Design review of the part built by this model. Coordinates are the model's own, in mm. A direction names the side the tool comes from. Round coordinates to 2 decimals unless told otherwise and drop trailing zeros. Write each loop counter-clockwise with the first axis right and the second up, starting at its lowest first coordinate (ties: lowest second). Pieces come first, ordered by that corner, then holes. Notation, with made-up numbers: M 21.5,45.25 L 30.5,45.25 A16 cw 30.5,53.25 Z; hole C -24.5,2 d6. An arc over 180 degrees is marked long. One line per question, with ' | ' between items. Start each with the question number.
Item 1: Add section D-D, the plane y = 13. State the section outline as (x, z) points.
Item 2: Draft analysis for pull direction X (two halves, no side actions). For faces 3 (the face through (6.82, 10.91, 29.4)), 4 (the face through (1.4, 6.4, 0.4)), 5 (the face through (4, -4, 31.75)), state which applies: released by +X, released by -X, zero draft, split by the parting line, or undercut.
Item 3: For L1, parallel to Z at x = 0, y = -7 (3 decimals); L2, parallel to Z at x = 0, y = 7.15 (3 decimals); L3, parallel to Y at x = 0, z = 17.5 (3 decimals), list the stretches that pass through material, from the lowest coordinate up.
Item 4: Add section A-A, the plane y = 0. Give the number of separate pieces and of enclosed holes in the cut face, and give its area (3 significant figures).
Item 5: Machinability: for faces 1 (the face through (11.4, 0.2, 26.988)), 2 (the face through (0.066, 7.023, 20.726)), which of the approach directions +Z, -Z, +X, -X, +Y, -Y give a long, thin tool a straight path to every point of the face, cutting with its end or side? Answer none if there is none.
Item 6: Insertion check: pin 1 Ø4 at (x, z) = (3, 5.5) entering from +Y; pin 2 Ø1 at (y, z) = (-10.5, 19) entering from -X; pin 3 Ø2 at (y, z) = (6, 21.5) entering from +X; pin 4 Ø5 at (x, z) = (0, 12.7) entering from -Y (3 decimals). Each pin has a flat end and moves straight along its axis. Give the tip position at first contact, or say it passes through.
Item 7: Add section C-C, the plane z = 12.7. State the section outline as (x, y) points (3 decimals).
```python
from build123d import *

# Parameters (mm, degrees)
SKETCH1_R               = 9.525
BOSS_EXTRUDE1_DEPTH     = 31.75
SKETCH18_R              = 17.4625
BOSS_EXTRUDE2_DEPTH     = 4.7625
SKETCH12_R              = 4.826
CUT_EXTRUDE3_DEPTH      = 31.75
CUT_EXTRUDE4_DEPTH      = 41.223628783
CUT_EXTRUDE4_DEPTH_BACK = 41.223628783
SKETCH14_R              = 1.5
SKETCH17_R              = 1.499997
CUT_EXTRUDE5_DEPTH      = 6.35
CIRPATTERN1_COUNT       = 3
FILLET1_R               = 1.5875


with BuildPart() as part:
    # Sketch1 → Boss-Extrude1 (new body)
    with BuildSketch(Plane.XY):
        Circle(SKETCH1_R)
    extrude(amount=BOSS_EXTRUDE1_DEPTH)

    # Sketch18 → Boss-Extrude2 (add)
    with BuildSketch(Plane.XY.offset(31.75)):
        Circle(SKETCH18_R)
    extrude(amount=-BOSS_EXTRUDE2_DEPTH)

    # Sketch12 → Cut-Extrude3 (cut)
    with BuildSketch(Plane(origin=(0, 0, 0), x_dir=(-1, 0, 0), z_dir=(0, 0, -1))):
        Circle(SKETCH12_R)
    extrude(amount=-CUT_EXTRUDE3_DEPTH, mode=Mode.SUBTRACT)

    # Sketch14 → Cut-Extrude4 (cut, two sides: drawn at the far end of the back side and taken through both)
    with BuildSketch(Plane(origin=(0, 0, 0), x_dir=(1, 0, 0), z_dir=(0, 1, 0)).offset(-CUT_EXTRUDE4_DEPTH_BACK)):
        with Locations(Location((0, -12.7, 0), (0, 0, 270))):
            Circle(SKETCH14_R)
        with Locations(Location((0, -22.225, 0), (0, 0, 270))):
            Circle(SKETCH14_R)
    extrude(amount=CUT_EXTRUDE4_DEPTH + CUT_EXTRUDE4_DEPTH_BACK, mode=Mode.SUBTRACT)

    # Sketch17 → Cut-Extrude5 (cut)
    with BuildSketch(Plane.XY.offset(31.75)):
        with Locations((7.14375, 12.373337957)):
            Circle(SKETCH17_R)
    cut_extrude5 = extrude(amount=-CUT_EXTRUDE5_DEPTH, mode=Mode.SUBTRACT)

    # CirPattern1: Cut-Extrude5 ×3 about axis
    cirpattern1_axis = Axis((0, 0, 0), (0, 0, 1))
    for i in range(1, CIRPATTERN1_COUNT):
        add(cut_extrude5.rotate(cirpattern1_axis, i * 360 / CIRPATTERN1_COUNT), mode=Mode.SUBTRACT)

    # Sketch16 → Cut-Revolve1 (revolve, cut)
    with BuildSketch(Plane(origin=(0, 0, 0), x_dir=(1, 0, 0), z_dir=(0, 1, 0))):
        Polygon((-6.35, 0), (-9.525, -6.35), (-9.525, 0), align=None)
    revolve(axis=Axis((0, 0, 0), (0, 0, 1)), mode=Mode.SUBTRACT)

    # Fillet1
    fillet1_edges = [part.edges().sort_by_distance(p)[0] for p in [
        (-9.525, 0, 26.9875),
    ]]
    fillet(fillet1_edges, radius=FILLET1_R)


solid = part.part
```
Computed values:
1) outline: M -11.66,26.99 L 5.78,26.99 L 5.78,31.75 L -11.66,31.75 Z; M 8.51,26.99 L 11.66,26.99 L 11.66,31.75 L 8.51,31.75 Z
2) face 3: undercut | face 4: split by the parting line | face 5: zero draft
3) L1: z = 1.3 to 11.2, 14.2 to 20.725, 23.725 to 31.75 | L2: z = 1.6 to 11.2, 14.2 to 20.725, 23.725 to 31.75 | L3: y = -9.525 to -4.826, 4.826 to 9.525
4) separate pieces: 3 | enclosed holes: 0 | area: 341 mm^2
5) face 1: -Z | face 2: +Y, -Y
6) pin 1: stops at y = 9.45 | pin 2: passes through | pin 3: stops at x = 8.11 | pin 4: stops at y = -9.525
7) outline: M -1.5,-9.406 L -1.5,-4.587 A4.826 cw -1.5,4.587 L -1.5,9.406 A9.525 ccw Z; M 1.5,-9.406 A9.525 ccw 1.5,9.406 L 1.5,4.587 A4.826 cw 1.5,-4.587 Z
